Autodesk Inventor part; units mm, degrees
ref_plane "YZ Plane" through (0, 0, 0) normal (1, 0, 0) x (0, 1, 0)
ref_plane "XZ Plane" through (0, 0, 0) normal (0, 1, 0) x (-1, 0, 0)
ref_plane "XY Plane" through (0, 0, 0) normal (0, 0, 1) x (1, 0, 0)
sketch "Sketch1" plane through (0, 0, 0) normal (0, 0, 1) x (1, 0, 0)
  circle A0 centre (0, 0) radius 6.75
  circle A1 centre (0, 0) radius 12
  dimension "d0" = 13.5
  dimension "d1" = 24
extrude "Extrusion1" add sketch "Sketch1" along normal blind 12.5
sketch "Sketch3" plane through (0, 0, 12.5) normal (0, 0, 1) x (1, 0, 0)
  circle A0 centre (0, 0) radius 10
  circle A1 centre (0, 0) radius 6.75
  dimension "d7" = 20
extrude "Extrusion3" add sketch "Sketch3" along normal blind 1
sketch "Sketch5" plane through (0, 0, 13.5) normal (0, 0, 1) x (1, 0, 0)
  line L0 (2, -8.55) -> (-2, -8.55)
  line L1 (-2, -8.55) -> (-2, -4.55)
  line L2 (-2, -4.55) -> (2, -4.55)
  line L3 (2, -4.55) -> (2, -8.55)
  line L4 (3.7816, -6.55) -> (-3.7816, -6.55)
  point P0 (0, 0)
  point P1 (0, -8.55)
  point P2 (-2, -6.55)
  point P3 (0, -6.55)
  dimension "d13" = 4
  dimension "d14" = 4
extrude "Extrusion5" cut sketch "Sketch5" against normal through all
properties part number "Outer Wheel Spacer"
Check sheet for the modelled part. Datum: model origin and axes. Units: mm. A direction names the side the tool comes from. Coordinates: 2 decimals unless noted, no trailing zeros. Order: outer loops, then holes, each group sorted by start corner. A loop starts at its lowest first (then second) coordinate and runs counter-clockwise, first axis right, second up. Notation, with made-up numbers: (-13, 75.25) -> (38, 75.25) arc R25 cw to (38, 101.25) -> close; hole circle Ø5 at (78.5, 65). An arc over 180 degrees is marked (long way). Write each question's results on one line, items separated by ' | '. Start each with the question number.
1) Section check B-B (z = 12). Enter the section's corners in (x, y).
2) Draft check along Y on faces 3 (the face through (-5, 9, 12.5)), 4 (the face through (-2.17, 9.76, 12.99)), 5 (the face through (2, -7, 7)). Enter one of: pulls with the +Y half, pulls with the -Y half, needs draft (parallel to the pull), parting line crosses it, or undercut.
3) Set-up check for faces 1 (the face through (-2, -8, 7)), 2 (the face through (5, -5, 0)): record each of +Z, -Z, +X, -X, +Y, -Y from which the full face is reachable in a straight line by a thin tool's end or side.
4) Depth check by flat-ended pin: pin 1 (4 mm diameter, centred on y = 4.5, z = 3.5, fed in from -X); pin 2 (1.2 mm diameter, centred on x = -1, z = 10, fed in from +Y); pin 3 (8 mm diameter, centred on y = 6, z = 8.5, fed in from -X); pin 4 (7 mm diameter, centred on x = 0, y = 0, fed in from +Z) (1 decimal). Enter the tip coordinate at first touch or a pass-through.
5) Section check A-A (y = 0). Enter the section's corners in (x, z), and give its area (3 significant figures).
6) Material ranges on line 1 along Y through (x, z) = (0, 7.75); line 2 along Z through (x, y) = (-3.25, 10.25); line 3 along X through (y, z) = (5.25, 2.25), recorded low to high.
7) Section check C-C (x = 0). Enter the section's corners in (y, z), and give its area (3 significant figures).
8) Section check D-D (x = 9.25). Enter the section's corners in (y, z).
Checked values:
1) outline: circle Ø24 at (0, 0); hole (-2, -8.55) -> (2, -8.55) -> (2, -6.45) arc R6.75 ccw (long way) to (-2, -6.45) -> close
2) face 3: needs draft | face 4: parting line crosses it | face 5: undercut
3) face 1: +Z, -Z | face 2: -Z, +X, -X, +Y, -Y
4) pin 1: x = -11.74 | pin 2: y = 11.99 | pin 3: x = -11.83 | pin 4: through
5) outline: (-12, 0) -> (-6.75, 0) -> (-6.75, 13.5) -> (-10, 13.5) -> (-10, 12.5) -> (-12, 12.5) -> close; (6.75, 0) -> (12, 0) -> (12, 12.5) -> (10, 12.5) -> (10, 13.5) -> (6.75, 13.5) -> close | area: 138 mm²
6) line 1: -12 to -8.55, 6.75 to 12 | line 2: 0 to 12.5 | line 3: -10.79 to -4.24, 4.24 to 10.79
7) outline: (-12, 0) -> (-8.55, 0) -> (-8.55, 13.5) -> (-10, 13.5) -> (-10, 12.5) -> (-12, 12.5) -> close; (6.75, 0) -> (12, 0) -> (12, 12.5) -> (10, 12.5) -> (10, 13.5) -> (6.75, 13.5) -> close | area: 113 mm²
8) outline: (-7.64, 0) -> (7.64, 0) -> (7.64, 12.5) -> (3.8, 12.5) -> (3.8, 13.5) -> (-3.8, 13.5) -> (-3.8, 12.5) -> (-7.64, 12.5) -> close
